Geometry: final body of the model. Coordinates: model frame, mm. A direction names the side the tool comes from. Round coordinates to 2 decimals unless told otherwise and drop trailing zeros. Write each loop counter-clockwise with the first axis right and the second up, starting at its lowest first coordinate (ties: lowest second). Pieces come first, ordered by that corner, then holes. Notation, with made-up numbers: (17.25, 38.5) -> (31.25, 38.5) arc R24 ccw to (31.25, 72.5) -> close; hole circle Ø1 at (86.5, 20.5). An arc over 180 degrees is marked (long way). Use one line per item in the form item = value. Start each with the question number.
1. Reachability of faces 4 (the face through (13.97, 23.564, 0.601)), 5 (the face through (-13.79, 23.21, 6.4)), 6 (the face through (13.42, -23.88, 6.4)), 7 (the face through (13.034, 7.424, 3.479)) from +Z, -Z, +X, -X, +Y, -Y: full face, straight path, thin tool, end or side. Return the list, or none.
2. Line query: L1, parallel to Y at x = -19, z = 2.25; L2, parallel to X at y = -19, z = 1.75; L3, parallel to X at y = -7, z = 4.75. Output: solid intervals per line, ascending.
3. Draft query along Y for faces 1 (the face through (32.68, -17.21, 3.45)), 2 (the face through (13.23, -24.63, 3.48)), 3 (the face through (-3, 11, 7)). Return one class per face: pulls with the +Y half, pulls with the -Y half, needs draft (parallel to the pull), parting line crosses it, or undercut.
4. Cut plane A-A, the plane x = 0. Return the cut outline in (y, z), plus the area to 3 significant figures.
5. Pin query (flat end, axial travel): pin 1 Ø2 at (x, z) = (-26.5, 6) entering from +Y; pin 2 Ø6 at (x, y) = (30.5, 4.5) entering from +Z; pin 3 Ø3 at (x, y) = (-32, -25) entering from -Z; pin 4 Ø3 at (y, z) = (22.5, 5) entering from -X. Return the tip coordinate at first contact, or that it passes through.
```python
from build123d import *

# Parameters (mm, degrees)
F0_R     = 11
F1_DEPTH = 7
F2_R     = 2


with BuildPart() as f1:
    # F0 (on Top) → F1 (new body)
    with BuildSketch(Plane.XY):
        with BuildLine():
            Line((-20.5688137101, -35.8657114123), (-6.0947750549, -13.7059737717))
            ThreePointArc((-6.0947750549, -13.7059737717), (0, -15), (6.0947750549, -13.7059737717))
            Line((6.0947750549, -13.7059737717), (20.5688137101, -35.8657114123))
            ThreePointArc((20.5688137101, -35.8657114123), (34.8857895537, -20.1413199897), (41.3450240629, 0.1197405075))
            Line((41.3450240629, 0.1197405075), (14.9171089973, 1.5747568579))
            ThreePointArc((14.9171089973, 1.5747568579), (12.9903810568, 7.5), (8.8223339424, 12.1312169138))
            Line((8.8223339424, 12.1312169138), (20.7762103528, 35.7459709048))
            ThreePointArc((20.7762103528, 35.7459709048), (0, 40.2826399794), (-20.7762103528, 35.7459709048))
            Line((-20.7762103528, 35.7459709048), (-8.8223339424, 12.1312169138))
            ThreePointArc((-8.8223339424, 12.1312169138), (-12.9903810568, 7.5), (-14.9171089973, 1.5747568579))
            Line((-14.9171089973, 1.5747568579), (-41.3450240629, 0.1197405075))
            ThreePointArc((-41.3450240629, 0.1197405075), (-34.8857895537, -20.1413199897), (-20.5688137101, -35.8657114123))
        make_face()
        with Locations((-22.5166604984, -13)):
            Circle(F0_R, mode=Mode.SUBTRACT)
        Circle(F0_R, mode=Mode.SUBTRACT)
        with Locations((22.5166604984, -13)):
            Circle(F0_R, mode=Mode.SUBTRACT)
        with Locations((0, 26)):
            Circle(F0_R, mode=Mode.SUBTRACT)
    extrude(amount=F1_DEPTH)

    # F2
    f2_edges = [f1.edges().sort_by_distance(p)[0] for p in [
        (-12.990381, 7.5, 7),
        (-14.799272, 23.938594, 7),
        (0, 40.28264, 7),
        (14.799272, 23.938594, 7),
        (12.990381, 7.5, 7),
        (28.131067, 0.847249, 7),
        (34.88579, -20.14132, 7),
        (13.331794, -24.785843, 7),
        (0, -15, 7),
        (-13.331794, -24.785843, 7),
        (-34.88579, -20.14132, 7),
        (-28.131067, 0.847249, 7),
        (0, 40.28264, 0),
        (-14.799272, 23.938594, 0),
        (14.799272, 23.938594, 0),
        (12.990381, 7.5, 0),
        (28.131067, 0.847249, 0),
        (13.331794, -24.785843, 0),
        (34.88579, -20.14132, 0),
        (-13.331794, -24.785843, 0),
        (0, -15, 0),
        (-34.88579, -20.14132, 0),
        (-28.131067, 0.847249, 0),
        (-12.990381, 7.5, 0),
    ]]
    fillet(f2_edges, radius=F2_R)


solid = f1.part
```
Outcome:
q1.face_4 = -Z, +X
q1.face_5 = +Z, -X
q1.face_6 = +Z, -Y
q1.face_7 = +Z, -Z, +X
q2.L1 = -33.46 to -23.42, -2.58 to 1.35, 32.24 to 36.52
q2.L2 = -35.51 to -31.74, -13.3 to -9.57, 9.57 to 13.3, 31.74 to 35.51
q2.L3 = -40.15 to -31.74, -13.3 to -8.49, 8.49 to 13.3, 31.74 to 40.15
q3.face_1 = undercut
q3.face_2 = pulls with the -Y half
q3.face_3 = needs draft
q4.outline = (-15, 2) arc R2 ccw to (-13, 0) -> (-11, 0) -> (-11, 7) -> (-13, 7) arc R2 ccw to (-15, 5) -> close; (11, 0) -> (15, 0) -> (15, 7) -> (11, 7) -> close; (37, 0) -> (38.28, 0) arc R2 ccw to (40.28, 2) -> (40.28, 5) arc R2 ccw to (38.28, 7) -> (37, 7) -> close
q4.area = 75.5 mm^2
q5.pin_1 = 0.96
q5.pin_2 = through
q5.pin_3 = 0.15
q5.pin_4 = -14.83
